Can you work these out from the drawing? Everything is in mm from the part's minimum corner. A direction names the side the tool comes from. Give positions to 0.01 mm unless a question says otherwise; leave off trailing zeros. Loops run counter-clockwise (first coordinate to the right, second up) from the corner with the lowest first, then second, coordinate; pieces in that order, holes last. Notation, with made-up numbers: (-20.75, 57.25) - (0.25, 57.25) arc R19 ccw to (0.25, 75.25) - close; hole circle Ø9 at (17.25, -36). An arc over 180 degrees is marked (long way). Answer in a Markdown table with one row per item.
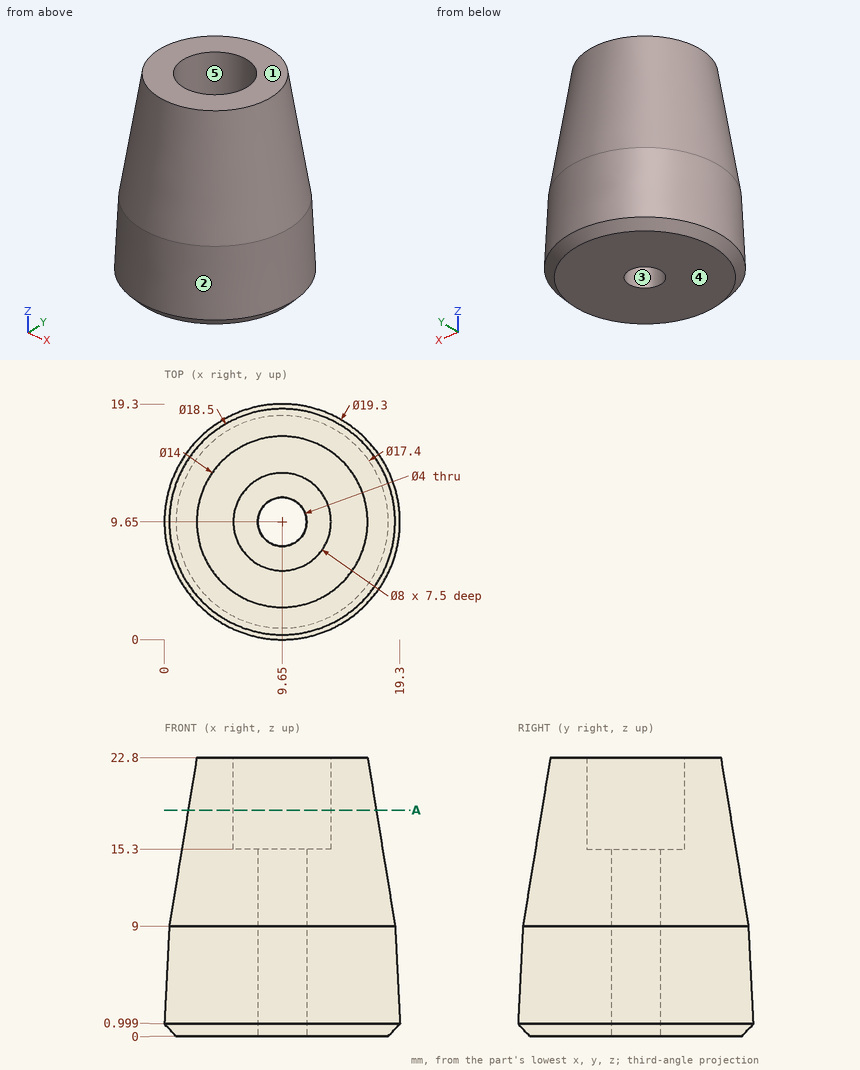
Q1. On a 3-axis mill with a long thin cutter (end or side, diameter ignored), from which of +Z, -Z, +X, -X, +Y, -Y can I reach the whole of each face in a straight line? I mean the marked faces 4 and 5. Say none if no direction works.
Checked values:
| item | result |
|---|---|
| face 4 | -Z, +X, -X, +Y, -Y |
| face 5 | +Z |
Q2. Imagine slicing it at A-A, the plane z = 18.5. Write out the boundary of the cut face in (x, y), and give its area (3 significant figures).
Checked values:
| item | result |
|---|---|
| outline | circle Ø15.4 at (9.65, 9.65); hole circle Ø8 at (9.65, 9.65) |
| area | 136 mm² |
Q3. For pin 1 (1.5 mm diameter, centred on y = 3.5, z = 5.5, fed in from +X); pin 2 (10 mm diameter, centred on x = 11.5, z = 14, fed in from +Y); pin 3 (1.5 mm diameter, centred on x = 7, z = 11.5, fed in from +Y); pin 4 (9 mm diameter, centred on x = 10.5, y = 9, fed in from +Z), each with a flat end and sliding along its axis, tell me the tip position at first contact or that it passes through.
Checked values:
| item | result |
|---|---|
| pin 1 | stops at x = 17.38 |
| pin 2 | stops at y = 18.86 |
| pin 3 | stops at y = 18.33 |
| pin 4 | stops at z = 22.8 |
Q4. If I drill on line 1 (Y direction, x = 11.5, z = 21) (1 decimal); line 2 (Y direction, x = 5.25, z = 15) (1 decimal); line 3 (Y direction, x = 10, z = 12.5), over which ranges is the centre line in solid material (lowest first)? Write a range as [from, to].
Checked values:
| item | result |
|---|---|
| line 1 | y = [2.6, 6.1], [13.2, 16.7] |
| line 2 | y = [2.6, 16.7] |
| line 3 | y = [0.98, 7.68], [11.62, 18.32] |
Q5. If we mould it in two halves opening along X, with no side actions, what happens to the marked faces 1, 2 and 3? For each: released by +X, released by -X, zero draft, split by the parting line, or undercut.
Checked values:
| item | result |
|---|---|
| face 1 | zero draft |
| face 2 | split by the parting line |
| face 3 | undercut |
